Input: part model. Units: mm. Frame: model coordinates. A direction names the side the tool comes from. Coordinates: 2 decimals unless noted, no trailing zeros. Loops run counter-clockwise (first coordinate to the right, second up) from the corner with the lowest first, then second, coordinate; pieces in that order, holes last. Notation, with made-up numbers: (2.5, -33.75) - (25.5, -33.75) arc R21 ccw to (25.5, -5.75) - close; hole circle Ø2 at (40.5, -3). An arc over 180 degrees is marked (long way). Use a Markdown table: item, result. Add a question column.
1. Section query D-D on z = 13. State how many separate pieces and enclosed holes the cut face has, then the cut area to 3 significant figures.
2. Section query A-A on z = 0. Return the cut outline in (x, y).
3. Ray query, L1, parallel to Z at x = 0, y = -28.3; L2, parallel to Z at x = 0, y = -6.5; L3, parallel to Y at x = 28, z = 14. Return the intervals inside material, ascending. Write a range as [from, to].
4. Section query B-B on x = 0. Return the cut outline in (y, z).
5. Draft query along X for faces 1 (the face through (24.015, -28.479, 13.066)), 2 (the face through (47.69, -13.8, 15.02)), 3 (the face through (-0.7, -30, 11.3)). Return one class per face: released by +X, released by -X, zero draft, split by the parting line, or undercut.
6. Contact query for flat-ended pins moving along their axis: P1, Ø6, axis at x = 11, y = -8.5, coming from the -Z side; P2, Ø8, axis at x = -30, y = -14.5, coming from the -Z side; P3, Ø4, axis at x = -22.52, z = 13, coming from the +Y side. Output: stop coordinate, or through.
7. Section query C-C on y = -16. Return the cut outline in (x, z).
8. Access query for faces 4 (the face through (-34, 0, -33)), 5 (the face through (10, -27, -10)). Directions: +Z, -Z, +X, -X, +Y, -Y. A direction counts if a zero-diameter tool reaches every point of the face in a straight line with its end or side. Return the directions, or none.
```python
from build123d import *

# Parameters (mm, degrees)
F0_R     = 50
F1_DEPTH = 30
F2_T     = -3
F3_R     = 2
F5_D     = 22
F7_D     = 3


with BuildPart() as f1:
    # F0 (on Front) → F1 (new body)
    with BuildSketch(Plane.XZ):
        Circle(F0_R)
    extrude(amount=F1_DEPTH)

    # F2
    f2_openings = [f1.faces().sort_by_distance(p)[0] for p in [
        (0, 0, 0),
    ]]
    offset(amount=F2_T, openings=f2_openings)

    # F3
    f3_edges = [f1.edges().sort_by_distance(p)[0] for p in [
        (-50, -30, 0),
    ]]
    fillet(f3_edges, radius=F3_R)

    # F5 (through all)
    with Locations(Plane.XZ.offset(30)):
        with Locations((0, 0)):
            Hole(F5_D / 2)

    # F7 (through all)
    with Locations(Plane.XZ.offset(30)):
        with Locations((0, -26), (-22.51666, 13), (22.51666, 13)):
            Hole(F7_D / 2)


solid = f1.part
```
Resolved:
| question | item | result |
|---|---|---|
| 1 | separate pieces | 3 |
| 1 | enclosed holes | 0 |
| 1 | area | 438 mm² |
| 2 | outline | (-50, -28) arc R2 ccw to (-48, -30) - (-11, -30) - (-11, -27) - (-47, -27) - (-47, 0) - (-50, 0) - close; (11, -30) - (48, -30) arc R2 ccw to (50, -28) - (50, 0) - (47, 0) - (47, -27) - (11, -27) - close |
| 3 | L1 | [-49.98, -27.5], [-24.5, -11], [11, 49.98] |
| 3 | L2 | [-50, -47], [47, 50] |
| 3 | L3 | [-30, -27] |
| 4 | outline | (-30, -48) arc R2 ccw to (-28, -50) - (0, -50) - (0, -47) - (-27, -47) - (-27, -27.5) - (-30, -27.5) - close; (-30, -24.5) - (-27, -24.5) - (-27, -11) - (-30, -11) - close; (-30, 11) - (-27, 11) - (-27, 47) - (0, 47) - (0, 50) - (-28, 50) arc R2 ccw to (-30, 48) - close |
| 5 | face 1 | undercut |
| 5 | face 2 | split by the parting line |
| 5 | face 3 | zero draft |
| 6 | P1 | z = -49.36 |
| 6 | P2 | z = -42.71 |
| 6 | P3 | y = -27 |
| 7 | outline | circle Ø100 at (0, 0); hole circle Ø94 at (0, 0) |
| 8 | face 4 | +Z, -Z, +X, -X, +Y |
| 8 | face 5 | +Y |
